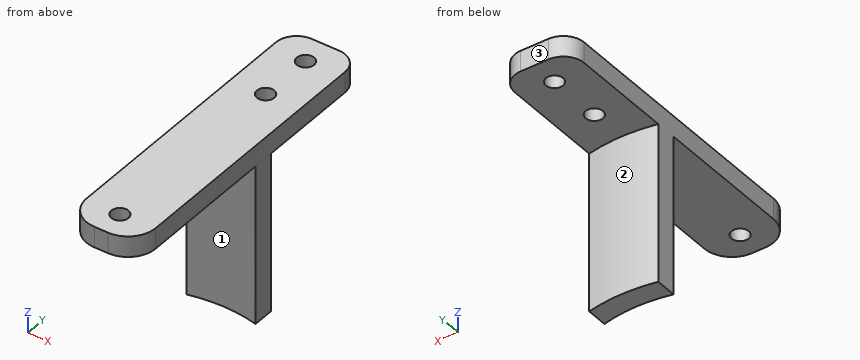
Autodesk Inventor part; units mm, degrees
ref_plane "YZ Plane" through (0, 0, 0) normal (1, 0, 0) x (0, 1, 0)
ref_plane "XZ Plane" through (0, 0, 0) normal (0, 1, 0) x (-1, 0, 0)
ref_plane "XY Plane" through (0, 0, 0) normal (0, 0, 1) x (1, 0, 0)
sketch "Sketch1" plane through (0, 0, 0) normal (0, 0, 1) x (1, 0, 0)
  line L0 (4, 0) -> (6, 0)
  line L1 (10, 4) -> (10, 42)
  line L2 (7, 45) -> (3, 45)
  line L3 (0, 42) -> (0, 4)
  arc A0 (0, 4) -> (4, 0) centre (4, 4) ccw
  arc A1 (6, 0) -> (10, 4) centre (6, 4) ccw
  arc A2 (3, 45) -> (0, 42) centre (3, 42) ccw
  arc A3 (10, 42) -> (7, 45) centre (7, 42) ccw
  point P0 (0, 0)
  point P1 (10, 45)
  point P2 (10, 0)
  point P3 (0, 45)
  dimension "d0" = 10
  dimension "d1" = 45
  dimension "d21" = 4
  dimension "d26" = 3
extrude "Extrusion1" add sketch "Sketch1" along normal blind 3
sketch "Sketch2" plane through (0, 0, 3) normal (0, 0, 1) x (1, 0, 0)
  circle A0 centre (5, 3.75) radius 1.25
  line L0 (0, 4) -> (0, 42)
  line L1 (6, 0) -> (4, 0)
  line L2 (3, 45) -> (7, 45)
  circle A1 centre (5, 33) radius 1.25
  circle A2 centre (5, 41) radius 1.25
  point P0 (0, 40)
  point P1 (0, 0)
  point P2 (10, 0)
  dimension "d4" = 2.5
  dimension "d14" = 3.75
  dimension "d18" = 5
  dimension "d27" = 2.5
  dimension "d28" = 2.5
  dimension "d29" = 4
  dimension "d30" = 8
extrude "Extrusion4" cut sketch "Sketch2" against normal through all
sketch "Sketch3" plane through (0, 0, 0) normal (0, 0, -1) x (-1, 0, 0)
  circle A0 centre (-5, 3.75) radius 1.25
  line L0 (-10, 4) -> (-10, 42)
  line L1 (0, 42) -> (0, 4)
  arc A1 (0, 24.0323) -> (-10, 24.0323) centre (-5, 3.75) ccw
  arc A2 (0, 27.1104) -> (-10, 27.1104) centre (-5, 3.75) ccw
  point P0 (-10, 40)
  point P1 (0, 40)
  point P2 (0, 0)
  dimension "d22" = 20.8895
  dimension "d23" = 3
extrude "Extrusion5" add sketch "Sketch3" along normal blind 23 contours L0 A2 L1 A1
equation "\"d4\" = centerHoleDia"
equation "\"d22\" = setScrewRingRad"
equation "\"d23\" = wallThickness"
equation "\"d24\" = wallHeight + wallThickness"
properties part number "arm"
Read the model definition and answer for the solid it produces. Units are mm, in the model's axes. Face numbers are marked on the shaded views. Give positions to 0.01 mm unless a question says otherwise; leave off trailing zeros. Write each loop counter-clockwise with the first axis right and the second up, starting at its lowest first coordinate (ties: lowest second). Pieces come first, ordered by that corner, then holes. Notation, with made-up numbers: (45.25, -7.75) - (89.25, -7.75) arc R13 ccw to (89.25, 10.25) - close; hole circle Ø9 at (24.25, 18). An arc over 180 degrees is marked (long way). Return JSON: item names as keys, results as strings.
Q1. A cutting plane is placed at C-C, the plane z = -5.5. Determine the outline of the cut face in (x, y).
Reply:
{"outline": "(0, 24.03) arc R20.89 cw to (10, 24.03) - (10, 27.11) arc R23.89 ccw to (0, 27.11) - close"}
Q2. For a pull along X with two mould halves and no side action, classify the marked faces 1, 2 and 3 as released by +X, released by -X, zero draft, split by the parting line, or undercut.
Reply:
{"face 1": "undercut", "face 2": "split by the parting line", "face 3": "zero draft"}
Q3. A cutting plane is placed at A-A, the plane y = 33. Determine the outline of the cut face in (x, z).
Reply:
{"outline": "(0, 0) - (3.75, 0) - (3.75, 3) - (0, 3) - close; (6.25, 0) - (10, 0) - (10, 3) - (6.25, 3) - close"}
Q4. A cutting plane is placed at D-D, the plane y = 23. Determine the outline of the cut face in (x, z).
Reply:
{"outline": "(0, 0) - (10, 0) - (10, 3) - (0, 3) - close"}
Q5. Consider line 1 along Y through (x, z) = (5, 1.4); line 2 along Z through (x, y) = (7.75, 31); line 3 along Y through (x, z) = (4.5, -10.5). Determine where each line is inside the solid, lowest interval first. Write a range as [from, to].
Reply:
{"line 1": "[0, 2.5], [5, 31.75], [34.25, 39.75], [42.25, 45]", "line 2": "[0, 3]", "line 3": "[24.63, 27.63]"}
Q6. Given P1, Ø6, axis at y = 31.5, z = -13.5, coming from the -X side; P2, Ø4, axis at x = 5, y = 41, coming from the -Z side; P3, Ø1, axis at x = 8.5, z = -14, coming from the -Y side, each flat-ended and moving along its own axis, determine where each tip first touches the part or whether it passes through.
Reply:
{"P1": "through", "P2": "z = 0", "P3": "y = 24.25"}
Q7. A cutting plane is placed at B-B, the plane x = 5. Determine the outline of the cut face in (y, z).
Reply:
{"outline": "(0, 0) - (2.5, 0) - (2.5, 3) - (0, 3) - close; (5, 0) - (24.64, 0) - (24.64, -23) - (27.64, -23) - (27.64, 0) - (31.75, 0) - (31.75, 3) - (5, 3) - close; (34.25, 0) - (39.75, 0) - (39.75, 3) - (34.25, 3) - close; (42.25, 0) - (45, 0) - (45, 3) - (42.25, 3) - close"}
